from build123d import *

# Parameters (mm, degrees)
SKETCH1_R           = 59
BOSS_EXTRUDE1_DEPTH = 3
SKETCH3_R           = 51.75
BOSS_EXTRUDE2_DEPTH = 10
SKETCH4_R           = 50
CUT_EXTRUDE2_DEPTH  = 10
SKETCH6_R           = 16
CUT_EXTRUDE4_DEPTH  = 15
SCALE1_SCALE        = 0.5


with BuildPart() as part:
    # Sketch1 → Boss-Extrude1 (new body)
    with BuildSketch(Plane(origin=(0, 0, 0), x_dir=(1, 0, 0), z_dir=(0, 1, 0))):
        with Locations(Location((0, 0, 0), (0, 0, 270))):
            Circle(SKETCH1_R)
    extrude(amount=BOSS_EXTRUDE1_DEPTH)

    # Sketch3 → Boss-Extrude2 (add)
    with BuildSketch(Plane(origin=(0, 3, 0), x_dir=(1, 0, 0), z_dir=(0, 1, 0))):
        with Locations(Location((0, 0, 0), (0, 0, 270))):
            Circle(SKETCH3_R)
    extrude(amount=BOSS_EXTRUDE2_DEPTH)

    # Sketch4 → Cut-Extrude2 (cut)
    with BuildSketch(Plane(origin=(0, 13, 0), x_dir=(1, 0, 0), z_dir=(0, 1, 0))):
        with Locations(Location((0, 0, 0), (0, 0, 270))):
            Circle(SKETCH4_R)
    extrude(amount=-CUT_EXTRUDE2_DEPTH, mode=Mode.SUBTRACT)

    # Sketch6 → Cut-Extrude4 (cut)
    with BuildSketch(Plane(origin=(0, 13, 0), x_dir=(1, 0, 0), z_dir=(0, 1, 0))):
        with Locations((2.110398292, -49.955442337)):
            Circle(SKETCH6_R)
    extrude(amount=-CUT_EXTRUDE4_DEPTH, mode=Mode.SUBTRACT)


with BuildPart() as part_1:
    # Scale1: scaled about (-0.143850324, 2.411415786, -3.405094959)
    add(part.part.scale(SCALE1_SCALE).moved(Location((-0.071925162, 1.205707893, -1.702547479))))


solid = part_1.part
Source: CAD feature listing. Evaluate the final solid. Frame: model axes, mm. A direction names the side the tool comes from. Round coordinates to 2 decimals unless told otherwise and drop trailing zeros. Loops run counter-clockwise (first coordinate to the right, second up) from the corner with the lowest first, then second, coordinate; pieces in that order, holes last. Notation, with made-up numbers: M 6.25,-40 L 37.25,-40 A16 cw 37.25,-21 Z; hole C 76.5,43 d4. An arc over 180 degrees is marked long. Return JSON: item names as keys, results as strings. Group by question number.
1. Pin query (flat end, axial travel): pin 1 (1 mm diameter, centred on y = 6.5, z = -4, fed in from -X); pin 2 (17.5 mm diameter, centred on x = 11, z = -5, fed in from +Y); pin 3 (1.5 mm diameter, centred on y = 6.5, z = -1, fed in from +X). Return the tip coordinate at first contact, or that it passes through.
2. Section query C-C on z = -10. Output: boundary loops of the cut face in (x, y).
3. Section query A-A on z = -2. Output: boundary loops of the cut face in (x, y).
4. Mould query, pull axis X, two halves, no side actions, for faces 3 (the face through (0, 2.706, -28)), 4 (the face through (-0.14, 5.171, -27.577)), 5 (the face through (0, 2.706, -3)). Classes: released by +X, released by -X, zero draft, split by the parting line, or undercut.
5. Reachability of faces 1 (the face through (0, 1.206, -2)), 2 (the face through (-0.14, 5.241, -26.702)) from +Z, -Z, +X, -X, +Y, -Y: full face, straight path, thin tool, end or side. Return the list, or none.
6. Material intervals for line 1 along Y through (x, z) = (-2, 11); line 2 along X through (y, z) = (3.25, -6); line 3 along X through (y, z) = (3.25, -17.5), sorted ascending. Write a range as from..to.
7. Section query B-B on x = -1.5. Output: boundary loops of the cut face in (y, z), and give its area (3 significant figures).
8. Section query D-D on y = 6. Output: boundary loops of the cut face in (x, z) (3 decimals).
Checks:
{
 "1": {"pin 1": "stops at x = -25.88", "pin 2": "stops at y = 2.71", "pin 3": "stops at x = 25.8"},
 "2": {"outline": "M -28.38,1.21 L 28.24,1.21 L 28.24,2.71 L 24.44,2.71 L 24.44,7.71 L 23.51,7.71 L 23.51,2.71 L -23.65,2.71 L -23.65,7.71 L -24.58,7.71 L -24.58,2.71 L -28.38,2.71 Z"},
 "3": {"outline": "M -29.57,1.21 L 29.43,1.21 L 29.43,2.71 L 25.8,2.71 L 25.8,7.71 L 24.93,7.71 L 24.93,2.71 L -25.07,2.71 L -25.07,7.71 L -25.95,7.71 L -25.95,2.71 L -29.57,2.71 Z"},
 "4": {"face 3": "zero draft", "face 4": "split by the parting line", "face 5": "undercut"},
 "5": {"face 1": "+Z, -Z, +X, -X, -Y", "face 2": "+Y"},
 "6": {"line 1": "y = 1.21..2.71", "line 2": "x = -25.59..-24.7, 24.56..25.44", "line 3": "x = -20.56..-19.45, 19.3..20.42"},
 "7": {"outline": "M 1.21,-31.17 L 2.71,-31.17 L 2.71,-27.54 L 7.71,-27.54 L 7.71,-26.66 L 2.71,-26.66 L 2.71,15.67 L 1.21,15.67 Z", "area": "74.6 mm²"},
 "8": {"outline": "M -7.017,23.223 A25.875 ccw long 8.95,22.549 A8 cw 8.819,21.663 A25 cw long -6.961,22.33 A8 cw Z"}
}
